Build history of the part. All positions in model axes, mm. A direction names the side the tool comes from. Coordinates: 2 decimals unless noted, no trailing zeros. Loops run counter-clockwise (first coordinate to the right, second up) from the corner with the lowest first, then second, coordinate; pieces in that order, holes last.
(1) Slice it at D-D (z = 16). Give the cut face in (x, y).
(2) Flat gauge pins, fed straight in: P1, Ø1.1, axis at x = 4, z = 12.5, coming from the -Y side; P2, Ø10, axis at y = -7, z = 12.5, coming from the +X side; P3, Ø5.5, axis at y = 0.5, z = 16.5, coming from the -X side; P4, Ø1.8, axis at x = 1, y = 10.5, coming from the +Z side. Where does each tip first touch, or does it go through?
(3) Slice it at A-A (y = 11). Give the cut face in (x, z), and give its area (3 significant figures).
(4) Tool access for faces 4 (the face through (4, 9.85, 13)), 5 (the face through (15, 0, 2)), 6 (the face through (-6, 0, 3)), 7 (the face through (0, -20, 2)): list every direction of +Z, -Z, +X, -X, +Y, -Y with a clear straight run to the whole face (end or side of a thin tool).
(5) Wall check: L1, parallel to Y at x = -10, z = 1; L2, parallel to Y at x = 1, z = 12.25; L3, parallel to Z at x = 17.5, y = 3.5. Give the ranges that are in metal, low to high.
(6) Slice it at B-B (y = 6). Give the cut face in (x, z), and give its area (3 significant figures).
(7) Two-plate mould, pull along X, no slides. Class faces 1 (the face through (-19.1, 19.14, 2.54)), 2 (the face through (4, -9.85, 13)), 3 (the face through (20, 0, 2)): pulls with the +X half, pulls with the -X half, needs draft (parallel to the pull), parting line crosses it, or undercut.
(8) Slice it at C-C (x = 8.5). Give the cut face in (y, z).
from build123d import *

# Parameters (mm, degrees)
SKETCH_W          = 40
SKETCH_H          = 40
SKETCH_W_2        = 8
SKETCH_H_2        = 28
SKETCH_W_3        = 9.4
SKETCH_H_3        = 13.4
PAD_DEPTH         = 5
SKETCH001_R       = 1.8
PAD001_DEPTH      = 17
POCKET_DEPTH      = 5
POCKET_DEPTH_BACK = -15
FILLET_R          = 3


with BuildPart() as part:
    # Sketch → Pad (new body)
    with BuildSketch(Plane.XY):
        Rectangle(SKETCH_W, SKETCH_H)
        with Locations((-11, 0)):
            Rectangle(SKETCH_W_2, SKETCH_H_2, mode=Mode.SUBTRACT)
        with Locations((11, 0)):
            Rectangle(SKETCH_W_2, SKETCH_H_2, mode=Mode.SUBTRACT)
        Rectangle(SKETCH_W_3, SKETCH_H_3, mode=Mode.SUBTRACT)
    extrude(amount=PAD_DEPTH)

    # Sketch001 (on Face18 of Pad) → Pad001 (join)
    with BuildSketch(Plane.XY.offset(5)):
        with BuildLine():
            Line((7, -14), (7, 14))
            ThreePointArc((7, 14), (0, 18.615773), (-7, 14))
            Line((-7, 14), (-7, -14))
            ThreePointArc((-7, -14), (0, -18.615773), (7, -14))
        make_face()
        with Locations((0, 11)):
            Circle(SKETCH001_R, mode=Mode.SUBTRACT)
        with Locations((0, -11)):
            Circle(SKETCH001_R, mode=Mode.SUBTRACT)
        with BuildLine():
            ThreePointArc((-3.305677, 9.85), (0, 7.5), (3.305677, 9.85))
            Line((3.305677, 9.85), (4.7, 9.85))
            Line((4.7, 9.85), (4.7, 0))
            Line((4.7, -9.85), (4.7, 0))
            Line((3.305677, -9.85), (4.7, -9.85))
            ThreePointArc((3.305677, -9.85), (0, -7.5), (-3.305677, -9.85))
            Line((-3.305677, -9.85), (-4.7, -9.85))
            Line((-4.7, -9.85), (-4.7, 0))
            Line((-4.7, 9.85), (-4.7, 0))
            Line((-3.305677, 9.85), (-4.7, 9.85))
        make_face(mode=Mode.SUBTRACT)
    extrude(amount=PAD001_DEPTH)

    # Sketch002 → Pocket (cut, two sides)
    with BuildSketch(Plane.YZ.offset(-4.7)) as pocket_sk:
        with BuildLine():
            ThreePointArc((-9.7, 0), (-7.57868, 0.87868), (-6.7, 3))
            Line((6.7, 3), (-6.7, 3))
            ThreePointArc((6.7, 3), (7.57868, 0.87868), (9.7, 0))
            Line((-9.7, 0), (9.7, 0))
        make_face()
    extrude(amount=-POCKET_DEPTH, mode=Mode.SUBTRACT)
    extrude(pocket_sk.sketch, amount=-POCKET_DEPTH_BACK, mode=Mode.SUBTRACT)

    # Fillet
    fillet_edges = [part.edges().sort_by_distance(p)[0] for p in [
        (20, 20, 2.5),
        (-20, 20, 2.5),
        (-20, -20, 2.5),
        (20, -20, 2.5),
    ]]
    fillet(fillet_edges, radius=FILLET_R)


solid = part.part
Response values:
1. outline: (-7, -14) arc R7.62 ccw to (7, -14) - (7, 14) arc R7.62 ccw to (-7, 14) - close; hole (-4.7, -9.85) - (-3.31, -9.85) arc R3.5 cw to (3.31, -9.85) - (4.7, -9.85) - (4.7, 9.85) - (3.31, 9.85) arc R3.5 cw to (-3.31, 9.85) - (-4.7, 9.85) - close; hole circle Ø3.6 at (0, -11); hole circle Ø3.6 at (0, 11)
2. P1: stops at y = -17.79
2. P2: stops at x = 7
2. P3: stops at x = -7
2. P4: stops at z = 22
3. outline: (-20, 0) - (-15, 0) - (-15, 5) - (-20, 5) - close; (-7, 0) - (7, 0) - (7, 22) - (1.8, 22) - (1.8, 5) - (-1.8, 5) - (-1.8, 22) - (-7, 22) - close; (15, 0) - (20, 0) - (20, 5) - (15, 5) - close
3. area: 297 mm2
4. face 4: +Z
4. face 5: +Z, -Z
4. face 6: -Z
4. face 7: +Z, -Z, +X, -X, -Y
5. L1: y = -20 to -14, 14 to 20
5. L2: y = -18.55 to -12.5, -9.5 to -7.65, 7.65 to 9.5, 12.5 to 18.55
5. L3: z = 0 to 5
6. outline: (-20, 0) - (-15, 0) - (-15, 5) - (-20, 5) - close; (-7, 3) - (-4.7, 3) - (-4.7, 22) - (-7, 22) - close; (4.7, 3) - (7, 3) - (7, 22) - (4.7, 22) - close; (15, 0) - (20, 0) - (20, 5) - (15, 5) - close
6. area: 137 mm2
7. face 1: pulls with the -X half
7. face 2: undercut
7. face 3: pulls with the +X half
8. outline: (-20, 0) - (-14, 0) - (-14, 5) - (-20, 5) - close; (14, 0) - (20, 0) - (20, 5) - (14, 5) - close
